Check sheet for the modelled part. Datum: model origin and axes. Units: mm. Face numbers are marked on the shaded views. A direction names the side the tool comes from. Give positions to 0.01 mm unless a question says otherwise; leave off trailing zeros. Order: outer loops, then holes, each group sorted by start corner. A loop starts at its lowest first (then second) coordinate and runs counter-clockwise, first axis right, second up.
from build123d import *

# Parameters (mm, degrees)
SKETCH1_R           = 11
SKETCH1_R_2         = 1.75
BOSS_EXTRUDE1_DEPTH = 8
SKETCH2_R           = 1.75
SKETCH2_R_2         = 5
BOSS_EXTRUDE2_DEPTH = 2
SKETCH3_R           = 1.75
SKETCH3_R_2         = 15.5
BOSS_EXTRUDE3_DEPTH = 10
SKETCH4_R           = 3
CUT_EXTRUDE1_DEPTH  = 15


with BuildPart() as part:
    # Sketch1 → Boss-Extrude1 (new body)
    with BuildSketch(Plane(origin=(0, 0, 0), x_dir=(1, 0, 0), z_dir=(0, 1, 0))):
        with BuildLine():
            Line((-15.5, 20.5), (15.5, 20.5))
            ThreePointArc((15.5, 20.5), (19.035533906, 19.035533906), (20.5, 15.5))
            Line((20.5, 15.5), (20.5, -15.5))
            ThreePointArc((20.5, -15.5), (19.035533906, -19.035533906), (15.5, -20.5))
            Line((15.5, -20.5), (-15.5, -20.5))
            ThreePointArc((-15.5, -20.5), (-19.035533906, -19.035533906), (-20.5, -15.5))
            Line((-20.5, -15.5), (-20.5, 15.5))
            ThreePointArc((-20.5, 15.5), (-19.035533906, 19.035533906), (-15.5, 20.5))
        make_face()
        Circle(SKETCH1_R, mode=Mode.SUBTRACT)
        with Locations((-15.5, 15.5)):
            Circle(SKETCH1_R_2, mode=Mode.SUBTRACT)
        with Locations((15.5, 15.5)):
            Circle(SKETCH1_R_2, mode=Mode.SUBTRACT)
        with Locations((15.5, -15.5)):
            Circle(SKETCH1_R_2, mode=Mode.SUBTRACT)
        with Locations((-15.5, -15.5)):
            Circle(SKETCH1_R_2, mode=Mode.SUBTRACT)
    extrude(amount=BOSS_EXTRUDE1_DEPTH)

    # Sketch2 → Boss-Extrude2 (add)
    with BuildSketch(Plane(origin=(0, 8, 0), x_dir=(1, 0, 0), z_dir=(0, 1, 0))):
        with BuildLine():
            Line((-20.5, 15.5), (-20.5, -15.5))
            ThreePointArc((-20.5, -15.5), (-19.035533906, -19.035533906), (-15.5, -20.5))
            Line((-15.5, -20.5), (15.5, -20.5))
            ThreePointArc((15.5, -20.5), (19.035533906, -19.035533906), (20.5, -15.5))
            Line((20.5, -15.5), (20.5, 15.5))
            ThreePointArc((20.5, 15.5), (19.035533906, 19.035533906), (15.5, 20.5))
            Line((15.5, 20.5), (-15.5, 20.5))
            ThreePointArc((-15.5, 20.5), (-19.035533906, 19.035533906), (-20.5, 15.5))
        make_face()
        with Locations((15.5, 15.5)):
            Circle(SKETCH2_R, mode=Mode.SUBTRACT)
        with Locations((15.5, -15.5)):
            Circle(SKETCH2_R, mode=Mode.SUBTRACT)
        with Locations((-15.5, 15.5)):
            Circle(SKETCH2_R, mode=Mode.SUBTRACT)
        Circle(SKETCH2_R_2, mode=Mode.SUBTRACT)
        with Locations((-15.5, -15.5)):
            Circle(SKETCH2_R, mode=Mode.SUBTRACT)
    extrude(amount=BOSS_EXTRUDE2_DEPTH)

    # Sketch3 → Boss-Extrude3 (add)
    with BuildSketch(Plane(origin=(0, 10, 0), x_dir=(1, 0, 0), z_dir=(0, 1, 0))):
        with BuildLine():
            Line((-20.5, 15.5), (-20.5, -15.5))
            ThreePointArc((-20.5, -15.5), (-19.035533906, -19.035533906), (-15.5, -20.5))
            Line((-15.5, -20.5), (15.5, -20.5))
            ThreePointArc((15.5, -20.5), (19.035533906, -19.035533906), (20.5, -15.5))
            Line((20.5, -15.5), (20.5, 15.5))
            ThreePointArc((20.5, 15.5), (19.035533906, 19.035533906), (15.5, 20.5))
            Line((15.5, 20.5), (-15.5, 20.5))
            ThreePointArc((-15.5, 20.5), (-19.035533906, 19.035533906), (-20.5, 15.5))
        make_face()
        with Locations((15.5, 15.5)):
            Circle(SKETCH3_R, mode=Mode.SUBTRACT)
        with Locations((15.5, -15.5)):
            Circle(SKETCH3_R, mode=Mode.SUBTRACT)
        with Locations((-15.5, -15.5)):
            Circle(SKETCH3_R, mode=Mode.SUBTRACT)
        with Locations((-15.5, 15.5)):
            Circle(SKETCH3_R, mode=Mode.SUBTRACT)
        Circle(SKETCH3_R_2, mode=Mode.SUBTRACT)
    extrude(amount=BOSS_EXTRUDE3_DEPTH)

    # Sketch4 → Cut-Extrude1 (cut)
    with BuildSketch(Plane(origin=(0, 20, 0), x_dir=(1, 0, 0), z_dir=(0, 1, 0))):
        with Locations((-15.5, 15.5)):
            Circle(SKETCH4_R)
        with Locations((15.5, 15.5)):
            Circle(SKETCH4_R)
        with Locations((15.5, -15.5)):
            Circle(SKETCH4_R)
        with Locations((-15.5, -15.5)):
            Circle(SKETCH4_R)
    extrude(amount=-CUT_EXTRUDE1_DEPTH, mode=Mode.SUBTRACT)


solid = part.part
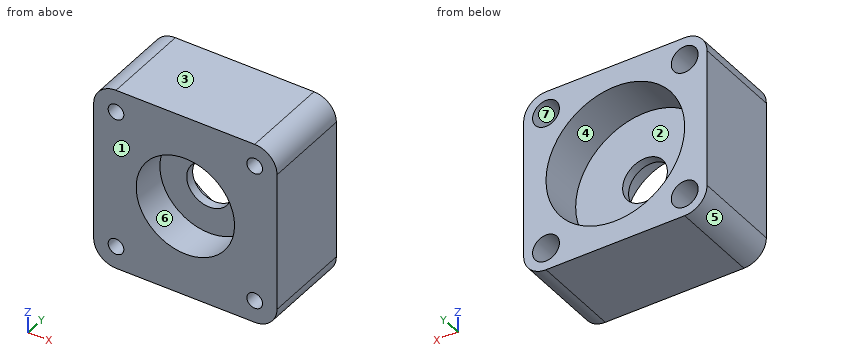
1) Section check B-B, the plane x = -2.5. Record the cut outline in (y, z), then the cut area to 3 significant figures.
Recorded:
outline: (0, -20.5) - (20, -20.5) - (20, -15.3) - (10, -15.3) - (10, -4.33) - (8, -4.33) - (8, -10.71) - (0, -10.71) - close; (0, 10.71) - (8, 10.71) - (8, 4.33) - (10, 4.33) - (10, 15.3) - (20, 15.3) - (20, 20.5) - (0, 20.5) - close
area: 325 mm2
2) Draft check along Z on the marked faces 1, 2, 3 and 4. Enter one of: +Z half, -Z half, draft (parallel to the pull), parting line (faces both ways), or undercut.
Recorded:
face 1: draft
face 2: undercut
face 3: +Z half
face 4: undercut
3) Section check A-A, the plane y = 18. Record the cut outline in (x, z), then the cut area to 3 significant figures.
Recorded:
outline: (-20.5, -15.5) arc R5 ccw to (-15.5, -20.5) - (15.5, -20.5) arc R5 ccw to (20.5, -15.5) - (20.5, 15.5) arc R5 ccw to (15.5, 20.5) - (-15.5, 20.5) arc R5 ccw to (-20.5, 15.5) - close; hole circle Ø6 at (-15.5, -15.5); hole circle Ø6 at (-15.5, 15.5); hole circle Ø31 at (0, 0); hole circle Ø6 at (15.5, -15.5); hole circle Ø6 at (15.5, 15.5)
area: 792 mm2
4) Depth check by flat-ended pin: pin 1 Ø2 at (x, z) = (-15.5, 15.5) entering from -Y; pin 2 Ø16 at (x, z) = (0, 0) entering from +Y; pin 3 Ø4 at (x, z) = (15.5, 15.5) entering from +Y. Enter the tip coordinate at first touch or a pass-through.
Recorded:
pin 1: passes through
pin 2: stops at y = 10
pin 3: stops at y = 5
5) Set-up check for the marked faces 5, 6 and 7: record each of +Z, -Z, +X, -X, +Y, -Y from which the full face is reachable in a straight line by a thin tool's end or side.
Recorded:
face 5: -Z, -X, +Y, -Y
face 6: -Y
face 7: +Y
6) Section check C-C, the plane z = 16. Record the cut outline in (x, y), then the cut area to 3 significant figures.
Recorded:
outline: (-20.47, 0) - (-17.18, 0) - (-17.18, 5) - (-18.46, 5) - (-18.46, 20) - (-20.47, 20) - close; (-13.82, 0) - (13.82, 0) - (13.82, 5) - (12.54, 5) - (12.54, 20) - (-12.54, 20) - (-12.54, 5) - (-13.82, 5) - close; (17.18, 0) - (20.47, 0) - (20.47, 20) - (18.46, 20) - (18.46, 5) - (17.18, 5) - close
area: 608 mm2
7) Section check D-D, the plane z = -1. Record the cut outline in (x, y), then the cut area to 3 significant figures.
Recorded:
outline: (-20.5, 0) - (-10.95, 0) - (-10.95, 8) - (-4.9, 8) - (-4.9, 10) - (-15.47, 10) - (-15.47, 20) - (-20.5, 20) - close; (4.9, 8) - (10.95, 8) - (10.95, 0) - (20.5, 0) - (20.5, 20) - (15.47, 20) - (15.47, 10) - (4.9, 10) - close
area: 316 mm2
8) Material ranges on L1, parallel to X at y = 9.75, z = -15.5; L2, parallel to X at y = 11, z = 17.5; L3, parallel to X at y = 17.5, z = 0, recorded low to high.
Recorded:
L1: x = -20.5 to -18.5, -12.5 to 12.5, 18.5 to 20.5
L2: x = -20.08 to -17.74, -13.26 to 13.26, 17.74 to 20.08
L3: x = -20.5 to -15.5, 15.5 to 20.5
